from build123d import *

# Parameters (mm, degrees)
SKETCH1_W            = 16
SKETCH1_H            = 1.5
BOSS_EXTRUDE1_DEPTH  = 22
FILLET1_R            = 2
SKETCH2_W            = 8
SKETCH2_H            = 2
BOSS_EXTRUDE2_DEPTH  = 0.25
SKETCH3_R            = 0.375
BOSS_EXTRUDE3_DEPTH  = 0.15
SKETCH4_R            = 0.3
BOSS_EXTRUDE4_DEPTH  = 8
BOSS_EXTRUDE5_DEPTH  = 8
SKETCH6_R            = 0.375
BOSS_EXTRUDE6_DEPTH  = 0.15
SKETCH7_W            = 16
SKETCH7_H            = 1.5
BOSS_EXTRUDE7_DEPTH  = 1.5
BOSS_EXTRUDE8_DEPTH  = 20.5
FILLET2_R            = 2
SKETCH9_W            = 14.259338364
SKETCH9_H            = 0.156424717
CUT_EXTRUDE1_DEPTH   = 20.5
SKETCH10_W           = 16
SKETCH10_H           = 20.335857824
SKETCH10_W_2         = 13.907599839
SKETCH10_H_2         = 18.335857824
BOSS_EXTRUDE9_DEPTH  = 10
SKETCH11_W           = 16
SKETCH11_H           = 20.335857824
BOSS_EXTRUDE10_DEPTH = 1
CUT_EXTRUDE2_DEPTH   = 11
SKETCH13_R           = 0.375
BOSS_EXTRUDE11_DEPTH = 25


with BuildPart() as part:
    # Sketch1 → Boss-Extrude1 (new body)
    with BuildSketch(Plane.XY):
        Rectangle(SKETCH1_W, SKETCH1_H)
    extrude(amount=BOSS_EXTRUDE1_DEPTH)

    # Fillet1
    fillet1_edges = [part.edges().sort_by_distance(p)[0] for p in [
        (-8, 0, 22),
        (8, 0, 22),
        (-8, 0, 0),
        (8, 0, 0),
    ]]
    fillet(fillet1_edges, radius=FILLET1_R)

    # Sketch2 → Boss-Extrude2 (add)
    with BuildSketch(Plane(origin=(0, 0, 0), x_dir=(-1, 0, 0), z_dir=(0, 0, -1))):
        with Locations((0, 0.5)):
            Rectangle(SKETCH2_W, SKETCH2_H)
    extrude(amount=BOSS_EXTRUDE2_DEPTH)

    # Sketch3 → Boss-Extrude3 (add)
    with BuildSketch(Plane(origin=(0, 0, -0.25), x_dir=(-1, 0, 0), z_dir=(0, 0, -1))):
        with Locations((-3, 0.5)):
            Circle(SKETCH3_R)
        Polygon((-3.05, 0.551330007), (-3.05, 0.800158256), (-2.95, 0.800158256), (-2.95, 0.551330007), (-2.7, 0.551330007), (-2.7, 0.45), (-2.95, 0.45), (-2.95, 0.2), (-3.05, 0.2), (-3.05, 0.45), (-3.3, 0.45), (-3.3, 0.551330007), align=None, mode=Mode.SUBTRACT)
        with Locations((0, 0.5)):
            Circle(SKETCH3_R)
        Polygon((-0.05, 0.2), (-0.05, 0.45), (-0.3, 0.45), (-0.3, 0.551330007), (-0.05, 0.551330007), (-0.05, 0.800158256), (0.05, 0.800158256), (0.05, 0.551330007), (0.3, 0.551330007), (0.3, 0.45), (0.05, 0.45), (0.05, 0.2), align=None, mode=Mode.SUBTRACT)
        with Locations((3, 0.5)):
            Circle(SKETCH3_R)
        Polygon((2.95, 0.2), (2.95, 0.45), (2.7, 0.45), (2.7, 0.551330007), (2.95, 0.551330007), (2.95, 0.800158256), (3.05, 0.800158256), (3.05, 0.551330007), (3.3, 0.551330007), (3.3, 0.45), (3.05, 0.45), (3.05, 0.2), align=None, mode=Mode.SUBTRACT)
    extrude(amount=BOSS_EXTRUDE3_DEPTH)

    # Sketch4 → Boss-Extrude4 (add)
    with BuildSketch(Plane(origin=(4, 0, 0), x_dir=(0, 0, -1), z_dir=(1, 0, 0))):
        with Locations((0.125, 1.7)):
            Circle(SKETCH4_R)
    extrude(amount=-BOSS_EXTRUDE4_DEPTH)

    # Sketch5 → Boss-Extrude5 (add)
    with BuildSketch(Plane(origin=(4, 0, 0), x_dir=(0, 0, -1), z_dir=(1, 0, 0))):
        Polygon((1.595306779, 3.344927555), (1.771017264, 3.168973693), (0.348913537, 1.749477894), (0.173440849, 1.924950583), align=None)
    extrude(amount=-BOSS_EXTRUDE5_DEPTH)

    # Sketch6 → Boss-Extrude6 (add)
    with BuildSketch(Plane(origin=(0, 0.701888086, 0.700600926), x_dir=(-1, 0, 0), z_dir=(0, -0.707755443, -0.706457524))):
        with Locations((3, 2.491187613)):
            Circle(SKETCH6_R)
        Polygon((2.95, 2.541187613), (2.95, 2.791187613), (3.05, 2.791187613), (3.05, 2.541187613), (3.3, 2.541187613), (3.3, 2.441187613), (3.05, 2.441187613), (3.05, 2.191187613), (2.95, 2.191187613), (2.95, 2.441187613), (2.7, 2.441187613), (2.7, 2.541187613), align=None, mode=Mode.SUBTRACT)
        with Locations((0, 2.491187613)):
            Circle(SKETCH6_R)
        Polygon((0.05, 2.441187613), (0.05, 2.191187613), (-0.05, 2.191187613), (-0.05, 2.441187613), (-0.3, 2.441187613), (-0.3, 2.541187613), (-0.05, 2.541187613), (-0.05, 2.791187613), (0.05, 2.791187613), (0.05, 2.541187613), (0.3, 2.541187613), (0.3, 2.441187613), align=None, mode=Mode.SUBTRACT)
        with Locations((-3, 2.491187613)):
            Circle(SKETCH6_R)
        Polygon((-2.95, 2.441187613), (-2.95, 2.191187613), (-3.05, 2.191187613), (-3.05, 2.441187613), (-3.3, 2.441187613), (-3.3, 2.541187613), (-3.05, 2.541187613), (-3.05, 2.791187613), (-2.95, 2.791187613), (-2.95, 2.541187613), (-2.7, 2.541187613), (-2.7, 2.441187613), align=None, mode=Mode.SUBTRACT)
    extrude(amount=BOSS_EXTRUDE6_DEPTH)

    # Sketch7 → Boss-Extrude7 (add)
    with BuildSketch(Plane(origin=(0, 0.877034448, 0.875869302), x_dir=(1, 0, 0), z_dir=(0, 0.707576635, 0.706636615))):
        with Locations((0, 2.622450086)):
            Rectangle(SKETCH7_W, SKETCH7_H)
    extrude(amount=BOSS_EXTRUDE7_DEPTH)

    # Sketch8 → Boss-Extrude8 (add)
    with BuildSketch(Plane(origin=(0, 2.383096713, -2.386266884), x_dir=(-1, 0, 0), z_dir=(0, 0.706636615, -0.707576635))):
        Polygon((-8, 1.239490402), (-4, 1.239490402), (4, 1.239490402), (8, 1.239490402), (8, 2.739490402), (-8, 2.739490402), align=None)
    extrude(amount=BOSS_EXTRUDE8_DEPTH)

    # Fillet2
    fillet2_edges = [part.edges().sort_by_distance(p)[0] for p in [
        (8, 2.730858715, 0.080944831),
        (-8, 2.730858715, 0.080944831),
        (8, 18.276864241, -15.485741141),
        (-8, 18.276864241, -15.485741141),
    ]]
    fillet(fillet2_edges, radius=FILLET2_R)

    # Sketch9 → Cut-Extrude1 (cut)
    with BuildSketch(Plane(origin=(0, 1.938399401, 1.935824224), x_dir=(1, 0, 0), z_dir=(0, 0.707576635, 0.706636615))):
        with Locations((0, 8.883775495)):
            Rectangle(SKETCH9_W, SKETCH9_H)
    extrude(amount=-CUT_EXTRUDE1_DEPTH, mode=Mode.SUBTRACT)

    # Sketch10 → Boss-Extrude9 (add)
    with BuildSketch(Plane(origin=(0, 0.877034448, 0.875869302), x_dir=(-1, 0, 0), z_dir=(0, -0.707576635, -0.706636615))):
        with Locations((-0.025561506, 13.721643007)):
            Rectangle(SKETCH10_W, SKETCH10_H)
        with Locations((-0.071761587, 13.721643007)):
            Rectangle(SKETCH10_W_2, SKETCH10_H_2, mode=Mode.SUBTRACT)
    extrude(amount=BOSS_EXTRUDE9_DEPTH)

    # Sketch11 → Boss-Extrude10 (add)
    with BuildSketch(Plane(origin=(0, -6.198731903, -6.190496846), x_dir=(-1, 0, 0), z_dir=(0, -0.707576635, -0.706636615))):
        with Locations((-0.025561506, 13.721643007)):
            Rectangle(SKETCH11_W, SKETCH11_H)
    extrude(amount=BOSS_EXTRUDE10_DEPTH)

    # Sketch12 → Cut-Extrude2 (cut)
    with BuildSketch(Plane.ZY.offset(7.974438494)):
        Polygon((-5.194715869, 6.939554806), (-11.745034119, 0.380522838), (-12.264104898, 0.898904028), (-5.713786648, 7.457935996), align=None)
    extrude(amount=-CUT_EXTRUDE2_DEPTH, mode=Mode.SUBTRACT)

    # Sketch13 → Boss-Extrude11 (add)
    with BuildSketch(Plane.ZY.offset(-8.025561506)):
        with Locations((-7.173250291, 5.474563224)):
            Circle(SKETCH13_R)
    extrude(amount=BOSS_EXTRUDE11_DEPTH)


solid = part.part
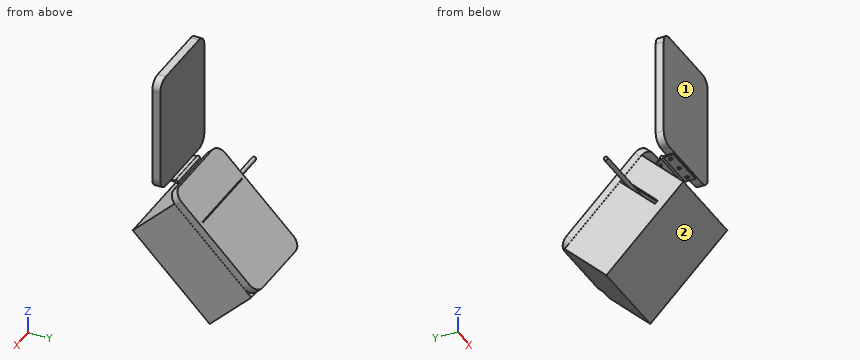
Design review of the part built by this model. Coordinates are the model's own, in mm. Face numbers are marked on the shaded views. A direction names the side the tool comes from. Give positions to 0.01 mm unless a question says otherwise; leave off trailing zeros. Return JSON: item names as keys, results as strings. Group by question number.
Item 1: Wall thickness on line 1 along X through (y, z) = (14.75, -15); line 2 along Z through (x, y) = (3.25, 0.5); line 3 along Z through (x, y) = (2.75, 5.5): over which ranges is each line inside the solid? List them lowest first.
Item 2: Clearance check with flat-ended pins moving along their axes: pin 1 Ø6 at (x, y) = (-1, 12.5) entering from -Z; pin 2 Ø0.5 at (x, y) = (3, 0.5) entering from -Z; pin 3 Ø5 at (x, y) = (4.5, 9.5) entering from +Z; pin 4 Ø5 at (x, y) = (1, 2) entering from -Z. State where each tip first meets the part, or that it passes through.
Item 3: Tool access review of the marked faces 1 and 2: name each direction out of +Z, -Z, +X, -X, +Y, -Y from which nothing blocks a thin tool from reaching the whole face with its end or side.
Return value:
{
 "1": {"line 1": "x = -7.97 to -6.88, 7.03 to 8.03", "line 2": "z = -14.31 to -12.9, -5.94 to -4.52, -0.25 to 22", "line 3": "z = -19.32 to -17.9, -7.55 to -6.8, -3.75 to -1.63"},
 "2": {"pin 1": "stops at z = -23.8", "pin 2": "stops at z = -14.56", "pin 3": "stops at z = -3.13", "pin 4": "stops at z = -18.32"},
 "3": {"face 1": "+Z, +X, -X, -Y", "face 2": "-Z, +X, -X, -Y"}
}
